Autodesk Inventor part; units mm, degrees
ref_plane "YZ Plane" through (0, 0, 0) normal (1, 0, 0) x (0, 1, 0)
ref_plane "XZ Plane" through (0, 0, 0) normal (0, 1, 0) x (-1, 0, 0)
ref_plane "XY Plane" through (0, 0, 0) normal (0, 0, 1) x (1, 0, 0)
sketch "Sketch1" plane through (0, 0, 0) normal (0, 0, 1) x (1, 0, 0)
  line L0 (0, 0) -> (142.24, 0)
  line L1 (142.24, 0) -> (142.24, 184.15)
  line L2 (142.24, 184.15) -> (0, 184.15)
  line L3 (0, 184.15) -> (0, 0)
  line L4 (4.3434, 179.8066) -> (137.8966, 179.8066)
  line L5 (137.8966, 179.8066) -> (137.8966, 4.3434)
  line L6 (137.8966, 4.3434) -> (4.3434, 4.3434)
  line L7 (4.3434, 4.3434) -> (4.3434, 179.8066)
  dimension "d0" = 184.15
  dimension "d1" = 142.24
  dimension "d2" = 4.3434
extrude "Extrusion1" add sketch "Sketch1" along normal blind 25.4
sketch "Sketch2" plane through (0, 0, 25.4) normal (0, 0, 1) x (1, 0, 0)
  line L0 (4.3434, 4.3434) -> (137.8966, 4.3434)
  line L1 (14.2875, 4.3434) -> (127.9525, 4.3434)
  line L2 (127.9525, 4.3434) -> (127.9525, 0)
  line L3 (127.9525, 0) -> (14.2875, 0)
  line L4 (14.2875, 0) -> (14.2875, 4.3434)
  line L5 (0, 184.15) -> (0, 0)
  line L6 (142.24, 0) -> (142.24, 184.15)
  dimension "d5" = 14.2875
  dimension "d6" = 14.2875
extrude "Extrusion2" cut sketch "Sketch2" against normal up to surface (25.4 mm away)
sketch "Sketch3" plane through (0, 0, 25.4) normal (0, 0, 1) x (1, 0, 0)
  line L0 (10.6934, 279.4) -> (17.0434, 279.4) construction
  line L1 (17.0434, 279.4) -> (17.0434, 25.4) construction
  line L2 (17.0434, 25.4) -> (10.6934, 25.4) construction
  line L3 (10.6934, 25.4) -> (10.6934, 279.4) construction
  line L4 (125.1966, 279.4) -> (131.5466, 279.4) construction
  line L5 (131.5466, 279.4) -> (131.5466, 25.4) construction
  line L6 (131.5466, 25.4) -> (125.1966, 25.4) construction
  line L7 (125.1966, 25.4) -> (125.1966, 279.4) construction
  line L8 (14.2875, 4.3434) -> (71.12, 4.3434) construction
  line L9 (71.12, 4.3434) -> (71.12, 0) construction
  line L10 (71.12, 0) -> (14.2875, 0) construction
  line L11 (14.2875, 0) -> (14.2875, 4.3434) construction
  line L12 (4.3434, 179.8066) -> (137.8966, 179.8066) construction
  line L13 (4.3434, 4.3434) -> (4.3434, 179.8066) construction
  line L14 (0, 0) -> (14.2875, 0) construction
  line L15 (137.8966, 179.8066) -> (137.8966, 4.3434) construction
  line L16 (127.9525, 0) -> (123.6091, 0) construction
  line L17 (123.6091, 0) -> (123.6091, -56.8325) construction
  line L18 (123.6091, -56.8325) -> (127.9525, -56.8325) construction
  line L19 (127.9525, -56.8325) -> (127.9525, 0) construction
  line L20 (137.8966, 4.3434) -> (112.4966, 4.3434) construction
  arc A0 (111.9446, 7.4193) -> (112.4966, 4.3434) centre (112.4966, 5.9309) ccw construction
  line L21 (111.9446, 7.4193) -> (137.8966, 17.0434) construction
  line L22 (137.8966, 4.3434) -> (137.8966, 179.8066) construction
  line L23 (159.3941, 36.0216) -> (266.702, 36.0216) construction
  line L24 (266.702, 36.0216) -> (266.702, 6.9446) construction
  line L25 (266.702, 6.9446) -> (159.3941, 6.9446) construction
  line L26 (159.3941, 6.9446) -> (159.3941, 36.0216) construction
  circle A1 centre (13.8684, 28.575) radius 3.175 construction
  circle A2 centre (128.3716, 28.575) radius 3.175 construction
  line L27 (42.7037, 4.3434) -> (12.0379, 25.9808)
  line L28 (111.3731, 7.0524) -> (130.6186, 26.3319)
  line L29 (111.0091, 5.3763) -> (123.6091, -28.4162)
  line L30 (63.5032, 17.7448) -> (103.5407, 17.7448) construction
  line L31 (103.5407, 17.7448) -> (103.5407, 7.0443) construction
  line L32 (103.5407, 7.0443) -> (63.5032, 7.0443) construction
  line L33 (63.5032, 7.0443) -> (63.5032, 17.7448) construction
  line L34 (144.8974, -10.3874) -> (251.178, -10.3874) construction
  line L35 (251.178, -10.3874) -> (251.178, -62.6009) construction
  line L36 (251.178, -62.6009) -> (144.8974, -62.6009) construction
  line L37 (144.8974, -62.6009) -> (144.8974, -10.3874) construction
  arc A3 (111.3731, 7.0524) -> (111.0091, 5.3763) centre (112.4966, 5.9309) ccw
  line L38 (3.9911, -9.0202) -> (42.7037, -9.0202) construction
  line L39 (42.7037, -9.0202) -> (42.7037, -18.258) construction
  line L40 (42.7037, -18.258) -> (3.9911, -18.258) construction
  line L41 (3.9911, -18.258) -> (3.9911, -9.0202) construction
  line L42 (8.6414, -30.8758) -> (98.6277, -30.8758) construction
  line L43 (98.6277, -30.8758) -> (98.6277, -107.8338) construction
  line L44 (98.6277, -107.8338) -> (8.6414, -107.8338) construction
  line L45 (8.6414, -107.8338) -> (8.6414, -30.8758) construction
  circle A4 centre (71.12, 145.5166) radius 17.5641 construction
  line L46 (33.02, 179.8066) -> (109.22, 179.8066) construction
  line L47 (109.22, 179.8066) -> (109.22, 173.4566) construction
  line L48 (109.22, 173.4566) -> (33.02, 173.4566) construction
  line L49 (33.02, 173.4566) -> (33.02, 179.8066) construction
  circle A5 centre (71.12, 145.5166) radius 25.4 construction
  point P0 (71.12, 179.8066)
  point P1 (71.12, 179.8066)
  point P2 (71.12, 173.4566)
  point P3 (71.12, 179.8066)
  dimension "d9" = 6.35
  dimension "d10" = 6.35
  dimension "d11" = 25.4
  dimension "d12" = 254
  dimension "d13" = 6.35
  dimension "d14" = 25.4
  dimension "d15" = 3.175
  dimension "d16" = 12.7
  dimension "d34" = 30.6658
  dimension "d35" = 21.6374
  dimension "d36" = 19.2795
  dimension "d37" = 19.2456
  dimension "d38" = 33.7925
  dimension "d39" = 12.6
  dimension "d40" = 35.1282
  dimension "d41" = 6.35
  dimension "d42" = 50.8
  dimension "d43" = 27.94
  dimension "d44" = 76.2
sketch "Sketch4" plane through (142.24, 0, 0) normal (1, 0, 0) x (0, 0, -1)
  line L0 (0, 4.3434) -> (-25.4, 4.3434)
  circle A0 centre (-19.05, 10.6934) radius 1.6129
  circle A1 centre (-6.35, 10.6934) radius 1.6129
  line L1 (-25.4, 17.0434) -> (-12.7, 4.3434) construction
  line L2 (0, 4.3434) -> (-25.4, 4.3434) construction
  line L3 (-12.7, 4.3434) -> (0, 17.0434) construction
  line L4 (0, 0) -> (0, 184.15) construction
  dimension "d17" = 3.2258
extrude "Extrusion3" cut sketch "Sketch4" against normal through all
pattern_linear "Rectangular Pattern1" count 13 spacing 12.7 along (0, 1, 0) of "Extrusion3"
sketch "Sketch6" plane through (0, 184.15, 0) normal (0, 1, 0) x (1, 0, 0)
  circle A0 centre (71.12, -6.35) radius 1.6129
  circle A1 centre (71.12, -19.05) radius 1.6129
  line L0 (142.24, 0) -> (0, 0)
  point P0 (71.12, 0)
  dimension "d23" = 3.2258
  dimension "d24" = 6.35
  dimension "d25" = 12.7
extrude "Extrusion4" cut sketch "Sketch6" against normal up to surface (4.3434 mm away)
pattern_linear "Rectangular Pattern2" count 3 spacing 12.7 along (-1, 0, 0) count 3 spacing -12.7 along (-1, 0, 0) of "Extrusion4"
equation "\"d6\" = d5"
equation "\"d13\" = d10"
properties part number "Bay Door Prototype Mk1"
Build history of the part. All positions in model axes, mm. A direction names the side the tool comes from. Coordinates: 2 decimals unless noted, no trailing zeros. Write each loop counter-clockwise with the first axis right and the second up, starting at its lowest first coordinate (ties: lowest second). Pieces come first, ordered by that corner, then holes.
(1) Pin check, flat tips, straight feed: pin 1 Ø3 at (x, z) = (45.72, 19.05) entering from -Y; pin 2 Ø4 at (y, z) = (48.79, 19.05) entering from -X; pin 3 Ø2 at (x, z) = (118, 19) entering from -Y. Stop position of each tip, or through.
(2) Cut at A-A on x = 10.5. List the corners of the cut face in (y, z).
(3) Cut at B-B on x = 25. List the corners of the cut face in (y, z), and give its area (3 significant figures).
(4) Drill centre lines: line 1 (Z direction, x = 58.42, y = 181.3); line 2 (X direction, y = 28, z = 15); line 3 (Y direction, x = 8, z = 15). Where is each one in solid material? Low to high.
(5) Mould opens along Y. For faces 1 (the flat face through (9, 4.343, 13)), 2 (the flat face through (137.897, 93, 13)), 3 (the flat face through (135, 0, 13)), 4 (the flat face through (14.288, 2, 13)) say: pulls with the +Y half, pulls with the -Y half, needs draft (parallel to the pull), parting line crosses it, or undercut.
(6) 3-axis set-ups, long thin cutter, end or side, ignore diameter. For faces 5 (the flat face through (127.952, 2, 13)), 6 (the flat face through (133, 4.343, 13)), 7 (the flat face through (7, 0, 13)): which of +Z, -Z, +X, -X, +Y, -Y reach the whole face in a straight line?
Working result:
1. pin 1: passes through
1. pin 2: stops at x = 0
1. pin 3: stops at y = 179.81
2. outline: (0, 0) - (4.34, 0) - (4.34, 25.4) - (0, 25.4) - close; (179.81, 0) - (184.15, 0) - (184.15, 25.4) - (179.81, 25.4) - close
3. outline: (179.81, 0) - (184.15, 0) - (184.15, 25.4) - (179.81, 25.4) - close
3. area: 110 mm2
4. line 1: z = 0 to 4.74, 7.96 to 17.44, 20.66 to 25.4
4. line 2: x = 0 to 4.34, 137.9 to 142.24
4. line 3: y = 0 to 4.34, 179.81 to 184.15
5. face 1: undercut
5. face 2: undercut
5. face 3: pulls with the -Y half
5. face 4: needs draft
6. face 5: +Z, -Z, -Y
6. face 6: +Z, -Z
6. face 7: +Z, -Z, +X, -X, -Y
